Job drawing, mm, ordinate dimensions from the low corner. One solid piece. Round coordinates to 2 decimals unless told otherwise and drop trailing zeros. Loops run counter-clockwise (first coordinate to the right, second up) from the corner with the lowest first, then second, coordinate; pieces in that order, holes last.
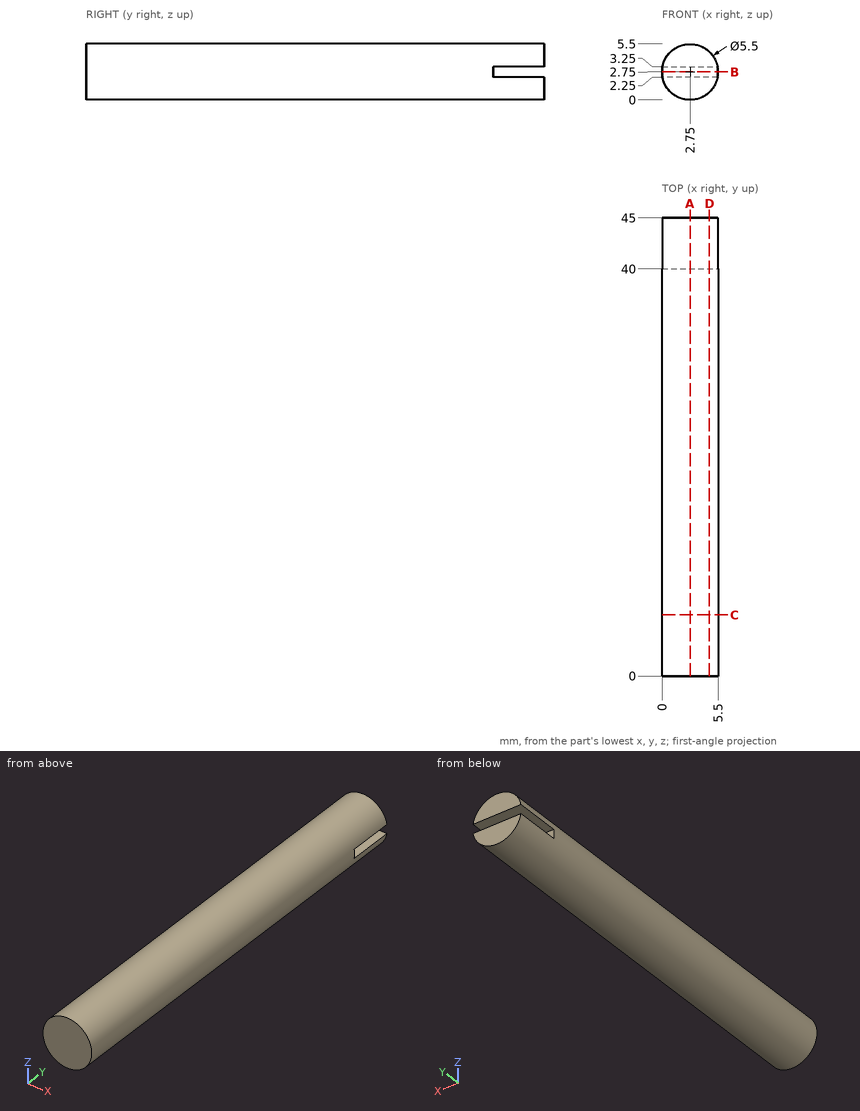
(1) Slice it at A-A on x = 2.75. List the corners of the cut face in (y, z).
Responses:
outline: (0, 0) - (45, 0) - (45, 2.25) - (40, 2.25) - (40, 3.25) - (45, 3.25) - (45, 5.5) - (0, 5.5) - close
(2) Slice it at B-B on z = 2.75. List the corners of the cut face in (x, y).
Responses:
outline: (0, 0) - (5.5, 0) - (5.5, 40) - (0, 40) - close
(3) Slice it at C-C on y = 6. List the corners of the cut face in (x, z), plus the area to 3 significant figures.
Responses:
outline: circle Ø5.5 at (2.75, 2.75)
area: 23.8 mm2
(4) Pin check, flat tip, straight feed: P1, Ø3, axis at y = 21.5, z = 4, coming from the +X side. Stop position of the tip, or through.
Responses:
P1: stops at x = 5.5
(5) Slice it at D-D on x = 4.65. List the corners of the cut face in (y, z).
Responses:
outline: (0, 0.76) - (45, 0.76) - (45, 2.25) - (40, 2.25) - (40, 3.25) - (45, 3.25) - (45, 4.74) - (0, 4.74) - close
(6) Probe line 1 (Y direction, x = 1.85, z = 2.5); line 2 (X direction, y = 28, z = 2.95); line 3 (Z direction, x = 2.2, y = 10.5). List the from-to ranges inside material, lowest first.
Responses:
line 1: y = 0 to 40
line 2: x = 0.01 to 5.49
line 3: z = 0.06 to 5.44
